The listing builds one solid part. Answer for the finished solid, in the listing's coordinates (mm). A direction names the side the tool comes from. Round coordinates to 2 decimals unless told otherwise and drop trailing zeros. Loops run counter-clockwise (first coordinate to the right, second up) from the corner with the lowest first, then second, coordinate; pieces in that order, holes last. Notation, with made-up numbers: M -2,-14 L 47,-14 A28 cw 47,18 Z; hole C 69,81 d3. An arc over 180 degrees is marked long. Answer as a JSON object with one key per item and string values.
```python
from build123d import *

# Parameters (mm, degrees)
SKETCH1_R           = 3
BOSS_EXTRUDE1_DEPTH = 40
SKETCH2_R           = 4
CUT_EXTRUDE1_DEPTH  = 40


with BuildPart() as part:
    # Sketch1 → Boss-Extrude1 (new body)
    with BuildSketch(Plane(origin=(0, 0, 0), x_dir=(0, 0, -1), z_dir=(1, 0, 0))):
        with BuildLine():
            Line((-24.097227121, 0), (-24.097227121, 5))
            Line((-24.097227121, 5), (-12.418356006, 5))
            Line((-12.418356006, 5), (-3.985022672, 28))
            Line((-3.985022672, 28), (9.902772879, 28))
            ThreePointArc((9.902772879, 28), (19.902772879, 38), (29.902772879, 28))
            Line((29.902772879, 28), (43.79056843, 28))
            Line((43.79056843, 28), (52.223901764, 5))
            Line((52.223901764, 5), (63.902772879, 5))
            Line((63.902772879, 5), (63.902772879, 0))
            Line((63.902772879, 0), (37.402772879, 0))
            Line((37.402772879, 0), (31.902772879, 15))
            Line((31.902772879, 15), (7.902772879, 15))
            Line((7.902772879, 15), (2.402772879, 0))
            Line((2.402772879, 0), (-24.097227121, 0))
        make_face()
        with Locations((19.902772879, 28)):
            Circle(SKETCH1_R, mode=Mode.SUBTRACT)
    extrude(amount=-BOSS_EXTRUDE1_DEPTH)

    # Sketch2 → Cut-Extrude1 (cut)
    with BuildSketch(Plane(origin=(0, 5, 0), x_dir=(1, 0, 0), z_dir=(0, 1, 0))):
        with Locations(Location((-20, -17.097227121, 0), (0, 0, 270))):
            Circle(SKETCH2_R)
        with Locations(Location((-20, 56.902772879, 0), (0, 0, 270))):
            Circle(SKETCH2_R)
    extrude(amount=-CUT_EXTRUDE1_DEPTH, mode=Mode.SUBTRACT)


solid = part.part
```
Item 1: Straight lines are drawn through the part: line 1 (Z direction, x = -35, y = 29); line 2 (X direction, y = 3.5, z = -54.5); line 3 (Y direction, x = -29, z = 13). For each, find the intervals that lie inside material, in ascending order.
Values follow:
{"line 1": "-29.85 to -22.73, -17.07 to -9.95", "line 2": "-40 to -23.2, -16.8 to 0", "line 3": "0 to 5"}
Item 2: The part is cut by section B-B (x = -30.5). Give the vertices of the cut face in (y, z).
Values follow:
{"outline": "M 0,-63.9 L 5,-63.9 L 5,-52.22 L 28,-43.79 L 28,-29.9 A10 ccw 28,-9.9 L 28,3.99 L 5,12.42 L 5,24.1 L 0,24.1 L 0,-2.4 L 15,-7.9 L 15,-31.9 L 0,-37.4 Z; hole C 28,-19.9 d6"}
Item 3: Determine the mould class of faces 6 (the face through (0, 19, -21)), 7 (the face through (-19.82, 2.54, -60.9)), 8 (the face through (-20, 0, 11)) for opening direction X: released by +X, released by -X, zero draft, split by the parting line, or undercut.
Values follow:
{"face 6": "released by +X", "face 7": "undercut", "face 8": "zero draft"}
Item 4: Which of the six approach directions +Z, -Z, +X, -X, +Y, -Y give full straight-line access (tool end or side, diameter ignored) to faces 1 (the face through (-19.72, 28.132, -16.906)), 2 (the face through (-20, 2, 24.097)), 3 (the face through (-19.72, 7.4, -34.69)), 4 (the face through (-20, 28, -3)), 5 (the face through (-20, 5, -62))?
Values follow:
{"face 1": "+X, -X", "face 2": "+Z, +X, -X, +Y, -Y", "face 3": "+X, -X, -Y", "face 4": "+Z, +X, -X, +Y", "face 5": "-Z, +X, -X, +Y"}
Item 5: The part is cut by section C-C (y = 10.5). Give the vertices of the cut face in (x, z).
Values follow:
{"outline": "M -40,-50.21 L 0,-50.21 L 0,-33.55 L -40,-33.55 Z; M -40,-6.25 L 0,-6.25 L 0,10.4 L -40,10.4 Z"}
Item 6: The part is cut by section D-D (z = -46). Give the vertices of the cut face in (x, y).
Values follow:
{"outline": "M -40,0 L 0,0 L 0,21.97 L -40,21.97 Z"}
Item 7: The part is cut by section A-A (x = -20). Give the vertices of the cut face in (y, z).
Values follow:
{"outline": "M 0,-63.9 L 5,-63.9 L 5,-60.9 L 0,-60.9 Z; M 0,-52.9 L 5,-52.9 L 5,-52.22 L 28,-43.79 L 28,-29.9 A10 ccw 28,-9.9 L 28,3.99 L 5,12.42 L 5,13.1 L 0,13.1 L 0,-2.4 L 15,-7.9 L 15,-31.9 L 0,-37.4 Z; M 0,21.1 L 5,21.1 L 5,24.1 L 0,24.1 Z; hole C 28,-19.9 d6"}
Item 8: Flat-ended cylindrical pins translate along their axes: P1, Ø4, axis at x = -20.5, z = -3.5, coming from the +Y side; P2, Ø5, axis at y = 28, z = -19.9, coming from the +X side; P3, Ø13, axis at x = -12.5, z = 20.5, coming from the +Y side; P4, Ø12, axis at x = -28, y = 32.5, coming from the +Z side (3 decimals). Find the tip coordinate at first contact, or state that the pin passes through.
Values follow:
{"P1": "y = 28", "P2": "through", "P3": "y = 5", "P4": "z = 4.535"}
